Geometry: see drawing. Coordinates: mm, zero at the bounding-box minimum. Round coordinates to 2 decimals unless told otherwise and drop trailing zeros. Loops run counter-clockwise (first coordinate to the right, second up) from the corner with the lowest first, then second, coordinate; pieces in that order, holes last.
(1) Mould query, pull axis Z, two halves, no side actions, for the marked faces 1, 2 and 3. Classes: pulls with the +Z half, pulls with the -Z half, needs draft (parallel to the pull), parting line crosses it, or undercut.
(2) Section A-A, the plane x = 10.75. Return the cut outline in (y, z) (3 decimals).
(3) Section C-C, the plane y = 1.75. Return the cut outline in (x, z).
(4) First-contact query: pin 1 Ø9.5 at (x, z) = (10, 20.5) entering from +Y; pin 2 Ø1.5 at (x, y) = (3.5, 1.5) entering from +Z. Flat tips, straight axial feed; report the tip coordinate or a pass-through.
(5) Material intervals for probe 1 along X at (y, z) = (6, 33); probe 2 along Z at (x, y) = (17.5, 3.5); probe 3 along Y at (x, z) = (15.5, 36.5), sorted ascending.
(6) Section B-B, the plane z = 39. Return the cut outline in (x, y) (3 decimals), plus the area to 3 significant figures.
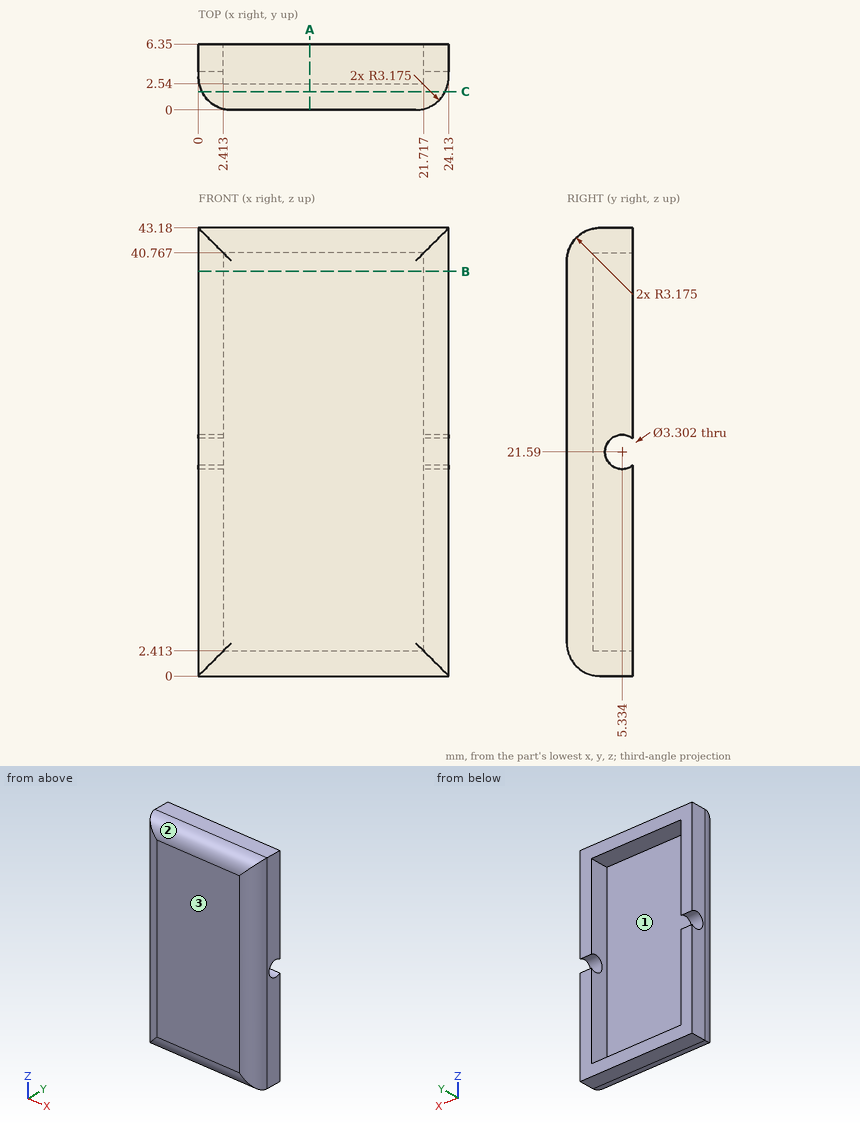
Output values:
1. face 1: undercut
1. face 2: pulls with the +Z half
1. face 3: needs draft
2. outline: (0, 3.175) arc R3.175 ccw to (3.175, 0) - (6.35, 0) - (6.35, 2.413) - (2.54, 2.413) - (2.54, 40.767) - (6.35, 40.767) - (6.35, 43.18) - (3.175, 43.18) arc R3.175 ccw to (0, 40.005) - close
3. outline: (0.34, 0.34) - (23.79, 0.34) - (23.79, 42.84) - (0.34, 42.84) - close
4. pin 1: stops at y = 2.54
4. pin 2: stops at z = 43.04
5. probe 1: x = 0 to 2.41, 21.72 to 24.13
5. probe 2: z = 0 to 2.41, 40.77 to 43.18
5. probe 3: y = 0 to 2.54
6. outline: (0, 3.175) arc R3.175 ccw to (3.175, 0) - (20.955, 0) arc R3.175 ccw to (24.13, 3.175) - (24.13, 6.35) - (21.717, 6.35) - (21.717, 2.54) - (2.413, 2.54) - (2.413, 6.35) - (0, 6.35) - close
6. area: 75.4 mm2
